from build123d import *

# Parameters (mm, degrees)
F0_R     = 2.5
F1_DEPTH = 9
F2_R     = 2.5
F3_DEPTH = 4
F4_R     = 5.25
F4_R_2   = 3.5
F5_DEPTH = 1.75
F6_R     = 0.7


with BuildPart() as f1:
    # F0 (on Front) → F1 (new body)
    with BuildSketch(Plane.XZ):
        with BuildLine():
            Line((22.3, 4.3), (22.3, 7.3))
            Line((22.3, 7.3), (0, 7.3))
            ThreePointArc((0, 7.3), (-7.3, 0), (0, -7.3))
            Line((0, -7.3), (22.3, -7.3))
            Line((22.3, -7.3), (22.3, -4.3))
            Line((22.3, -4.3), (14.3, -4.3))
            ThreePointArc((14.3, -4.3), (10, 0), (14.3, 4.3))
            Line((14.3, 4.3), (22.3, 4.3))
        make_face()
        Circle(F0_R, mode=Mode.SUBTRACT)
    extrude(amount=F1_DEPTH)

    # F2 (on face) → F3 (cut)
    with BuildSketch(Plane.XZ.offset(9)):
        Polygon((4.125, -2.38157), (4.125, 2.38157), (0, 4.76314), (-4.125, 2.38157), (-4.125, -2.38157), (0, -4.76314), align=None)
        Circle(F2_R, mode=Mode.SUBTRACT)
    extrude(amount=-F3_DEPTH, mode=Mode.SUBTRACT)

    # F4 (on Front) → F5 (cut)
    with BuildSketch(Plane.XZ):
        Circle(F4_R)
        Circle(F4_R_2, mode=Mode.SUBTRACT)
    extrude(amount=F5_DEPTH, mode=Mode.SUBTRACT)

    # F6
    f6_edges = [f1.edges().sort_by_distance(p)[0] for p in [
        (-5.25, -1.75, 0),
        (-3.5, -1.75, 0),
    ]]
    fillet(f6_edges, radius=F6_R)


solid = f1.part
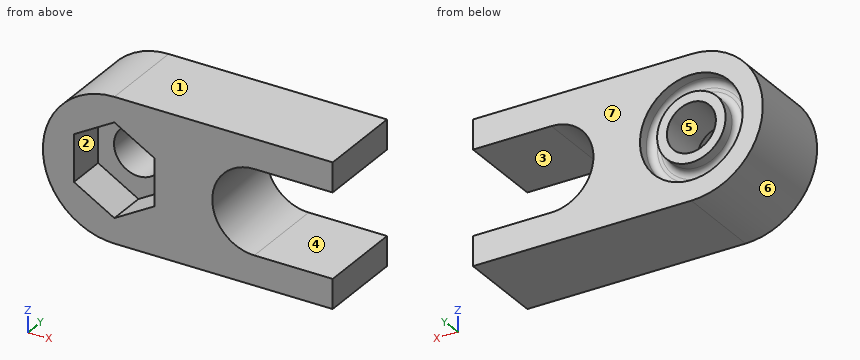
Design review of the part built by this model. Coordinates are the model's own, in mm. Face numbers are marked on the shaded views. A direction names the side the tool comes from. Round coordinates to 2 decimals unless told otherwise and drop trailing zeros. Write each loop counter-clockwise with the first axis right and the second up, starting at its lowest first coordinate (ties: lowest second). Pieces come first, ordered by that corner, then holes.
Item 1: For the marked faces 1, 2 and 3, list the 3-axis set-ups (+Z, -Z, +X, -X, +Y, -Y) from which the entire face can be reached by the end or side of a thin tool; tool diameter is ignored.
Item 2: Draft analysis for pull direction Z (two halves, no side actions). For the marked faces 4, 5, 6 and 7, state which applies: released by +Z, released by -Z, zero draft, split by the parting line, or undercut.
Item 3: Wall thickness on L1, parallel to Z at x = 0, y = -0.65; L2, parallel to Z at x = 15.25, y = -5; L3, parallel to Z at x = 12, y = -8.25: over which ranges is each line inside the solid? List them lowest first.
Item 4: Consider section B-B on y = -3. Give the boundary of the cut face in (x, z), and give its area (3 significant figures).
Item 5: For pin 1 Ø4 at (x, z) = (-1, -1.5) entering from -Y; pin 2 Ø3 at (y, z) = (-8, -1) entering from +X; pin 3 Ø2 at (y, z) = (-5.5, 4.5) entering from -X, all flat-tipped, find the tip position at first contact; note any pin that passes through.
Item 6: Consider section D-D on y = -5.75. Give the boundary of the cut face in (x, z) (3 decimals), and give its area (4 significant figures).
Item 7: Consider section A-A on z = 0. Give the boundary of the cut face in (x, y) (3 decimals).
Item 8: Consider section C-C on x = 20. Give the boundary of the cut face in (y, z), and give its area (3 significant figures).
Check values:
1. face 1: +Z, +X, -X, +Y, -Y
1. face 2: -Y
1. face 3: +X, +Y, -Y
2. face 4: undercut
2. face 5: undercut
2. face 6: split by the parting line
2. face 7: zero draft
3. L1: z = -7.3 to -5.25, -3.5 to -2.5, 2.5 to 3.5, 5.25 to 7.3
3. L2: z = -7.3 to -4.3, 4.3 to 7.3
3. L3: z = -7.3 to -3.63, 3.63 to 7.3
4. outline: (0, -7.3) - (22.3, -7.3) - (22.3, -4.3) - (14.3, -4.3) arc R4.3 cw to (14.3, 4.3) - (22.3, 4.3) - (22.3, 7.3) - (0, 7.3) arc R7.3 ccw to start; hole circle Ø5 at (0, 0)
4. area: 292 mm2
5. pin 1: stops at y = -5
5. pin 2: stops at x = 10.8
5. pin 3: stops at x = -6.41
6. outline: (0, -7.3) - (22.3, -7.3) - (22.3, -4.3) - (14.3, -4.3) arc R4.3 cw to (14.3, 4.3) - (22.3, 4.3) - (22.3, 7.3) - (0, 7.3) arc R7.3 ccw to start; hole (-4.125, -2.382) - (0, -4.763) - (4.125, -2.382) - (4.125, 2.382) - (0, 4.763) - (-4.125, 2.382) - close
6. area: 252.5 mm2
7. outline: (-7.3, -9) - (-4.125, -9) - (-4.125, -5) - (-2.5, -5) - (-2.5, 0) - (-3.5, 0) - (-3.5, -1.05) arc R0.7 cw to (-4.2, -1.75) - (-4.55, -1.75) arc R0.7 cw to (-5.25, -1.05) - (-5.25, 0) - (-7.3, 0) - close; (2.5, -5) - (4.125, -5) - (4.125, -9) - (10, -9) - (10, 0) - (5.25, 0) - (5.25, -1.05) arc R0.7 cw to (4.55, -1.75) - (4.2, -1.75) arc R0.7 cw to (3.5, -1.05) - (3.5, 0) - (2.5, 0) - close
8. outline: (-9, -7.3) - (0, -7.3) - (0, -4.3) - (-9, -4.3) - close; (-9, 4.3) - (0, 4.3) - (0, 7.3) - (-9, 7.3) - close
8. area: 54.0 mm2
